```python
from build123d import *

# Parameters (mm, degrees)
ESTRUSIONE_ESTRUSIONE1_DEPTH       = 5.1
FORO_FILETTATO_M3X0_5_1_AT_2_COUNT = 2
FORO_FILETTATO_M3X0_5_1_AT_2_PITCH = 14


with BuildPart() as part:
    # Schizzo1 → Estrusione-Estrusione1 (new body)
    with BuildSketch(Plane.XY):
        with BuildLine():
            Line((37.65394009, 53.683010839), (17.60394009, 53.683010839))
            Line((17.60394009, 53.683010839), (17.60394009, 48.851504979))
            add(Edge.make_bspline(
                [(21.317368868, 46.227364164), (20.952056874, 47.845897177), (19.207385128, 48.898989615), (17.60394009, 48.851504979)],
                knots=[0, 0, 0, 0, 1, 1, 1, 1], degree=3))
            Line((21.317368868, 46.227364164), (21.317368868, 24.338657514))
            add(Edge.make_bspline(
                [(21.317368868, 24.338657514), (20.952056874, 22.720124501), (19.207385128, 21.667032063), (17.60394009, 21.714516699)],
                knots=[0, 0, 0, 0, 1, 1, 1, 1], degree=3))
            Line((17.60394009, 21.714516699), (17.60394009, 16.883010839))
            Line((17.60394009, 16.883010839), (37.65394009, 16.883010839))
            Line((37.65394009, 16.883010839), (37.65394009, 21.714516699))
            add(Edge.make_bspline(
                [(33.940511311, 24.338657514), (34.305823306, 22.720124501), (36.050495052, 21.667032063), (37.65394009, 21.714516699)],
                knots=[0, 0, 0, 0, 1, 1, 1, 1], degree=3))
            Line((33.940511311, 24.338657514), (33.940511311, 46.227364164))
            add(Edge.make_bspline(
                [(33.940511311, 46.227364164), (34.305823306, 47.845897177), (36.050495052, 48.898989615), (37.65394009, 48.851504979)],
                knots=[0, 0, 0, 0, 1, 1, 1, 1], degree=3))
            Line((37.65394009, 48.851504979), (37.65394009, 53.683010839))
        make_face()
        with BuildLine():
            ThreePointArc((25.92894009, 43.033010839), (27.62894009, 44.733010839), (29.32894009, 43.033010839))
            Line((29.32894009, 43.033010839), (29.32894009, 27.533010839))
            ThreePointArc((29.32894009, 27.533010839), (27.62894009, 25.833010839), (25.92894009, 27.533010839))
            Line((25.92894009, 27.533010839), (25.92894009, 43.033010839))
        make_face(mode=Mode.SUBTRACT)
    extrude(amount=ESTRUSIONE_ESTRUSIONE1_DEPTH)

    # Schizzo2 → Foro filettato M3x0.5-1 (revolve, cut)
    with BuildSketch(Plane(origin=(20.62894009, 53.683010839, 2.55), x_dir=(0, 0, 1), z_dir=(1, 0, 0))):
        Polygon((0, 0), (0, 8.751075774), (1.25, 8), (1.25, 0), align=None)
    foro_filettato_m3x0_5_1 = revolve(axis=Axis((20.62894009, 60.033010839, 2.55), (0, -1, 0)), mode=Mode.SUBTRACT)

    # Foro filettato M3x0.5-1 at 2: Foro filettato M3x0.5-1 ×2
    with Locations(*[(i * FORO_FILETTATO_M3X0_5_1_AT_2_PITCH, 0, 0) for i in range(1, FORO_FILETTATO_M3X0_5_1_AT_2_COUNT)]):
        add(foro_filettato_m3x0_5_1, mode=Mode.SUBTRACT)

    # Specchia1: Foro filettato M3x0.5-1 across plane
    add(foro_filettato_m3x0_5_1.mirror(Plane.ZX.offset(35.283010839)), mode=Mode.SUBTRACT)

    # Specchia1 copy 1 sketch → Specchia1 copy 1 (revolve, cut)
    with BuildSketch(Plane(origin=(34.62894009, 16.883010839, 2.55), x_dir=(0, 0, 1), z_dir=(1, 0, 0))):
        Polygon((0, 0), (0, -8.751075774), (1.25, -8), (1.25, 0), align=None)
    revolve(axis=Axis((34.62894009, 10.533010839, 2.55), (0, -1, 0)), mode=Mode.SUBTRACT)


solid = part.part
```
The model under review builds one solid part; all positions refer to its coordinate system, in mm. A direction names the side the tool comes from. Give positions to 0.01 mm unless a question says otherwise; leave off trailing zeros. Write each loop counter-clockwise with the first axis right and the second up, starting at its lowest first coordinate (ties: lowest second). Pieces come first, ordered by that corner, then holes. Notation, with made-up numbers: (-2, 16) - (33, 16) arc R31 cw to (33, 43) - close; hole circle Ø2 at (43.25, 2.5). An arc over 180 degrees is marked (long way). Answer in a Markdown table with one row per item. Add a question column.
1. Tool access review of faces 5 (the cylindrical face through (27.666, 25.833, 2.514)), 6 (the cylindrical face through (33.39, 19.94, 2.39)), 7 (the cylindrical face through (21.85, 50.63, 2.28)), 8 (the flat face through (33.941, 35, 3)): name each direction out of +Z, -Z, +X, -X, +Y, -Y from which nothing blocks a thin tool from reaching the whole face with its end or side.
2. Wall thickness on line 1 along X through (y, z) = (49, 2.55); line 2 along X through (y, z) = (33, 4.25); line 3 along Y through (x, z) = (28.25, 2.5): over which ranges is each line inside the solid? List them lowest first. Write a range as [from, to].
3. We need section A-A on y = 36.5. Write out the cut boundary in (x, z).
4. We need section B-B on z = 2.55. State how many separate pieces and enclosed holes the cut face has, then the cut area to 3 significant figures.
5. Draft analysis for pull direction X (two halves, no side actions). For faces 1 (the flat face through (17.604, 19, 3)), 2 (the cylindrical face through (33.39, 50.63, 2.39)), 3 (the flat face through (37.654, 19, 3)), 4 (the flat face through (29.329, 35, 3)), state which applies: +X half, -X half, draft (parallel to the pull), parting line (faces both ways), or undercut.
6. Insertion check: P1, Ø1.5, axis at x = 34.63, z = 2.55, coming from the -Y side; P2, Ø1.5, axis at y = 33.5, z = 3.5, coming from the -X side; P3, Ø3, axis at y = 47, z = 4.5, coming from the -X side. Each pin has a flat end and moves straight along its axis. Give the tip position at first contact, or say it passes through.
Ans:
| question | item | result |
|---|---|---|
| 1 | face 5 | +Z, -Z |
| 1 | face 6 | -Y |
| 1 | face 7 | +Y |
| 1 | face 8 | +Z, -Z, +X |
| 2 | line 1 | x = [17.6, 19.38], [21.88, 33.38], [35.88, 37.65] |
| 2 | line 2 | x = [21.32, 25.93], [29.33, 33.94] |
| 2 | line 3 | y = [16.88, 25.95], [44.62, 53.68] |
| 3 | outline | (21.32, 0) - (25.93, 0) - (25.93, 5.1) - (21.32, 5.1) - close; (29.33, 0) - (33.94, 0) - (33.94, 5.1) - (29.33, 5.1) - close |
| 4 | separate pieces | 5 |
| 4 | enclosed holes | 1 |
| 4 | area | 420 mm^2 |
| 5 | face 1 | -X half |
| 5 | face 2 | undercut |
| 5 | face 3 | +X half |
| 5 | face 4 | undercut |
| 6 | P1 | stops at y = 25.18 |
| 6 | P2 | stops at x = 21.32 |
| 6 | P3 | stops at x = 19.32 |
